Here's how the part is built. I have some questions about the finished solid (model axes, mm). Coordinates: 2 decimals unless noted, no trailing zeros. Write each loop counter-clockwise with the first axis right and the second up, starting at its lowest first coordinate (ties: lowest second). Pieces come first, ordered by that corner, then holes.
```python
from build123d import *

# Parameters (mm, degrees)
SKIZZE1_W                       = 8
SKIZZE1_H                       = 16
AUFSATZ_LINEAR_AUSTRAGEN1_DEPTH = 4.7
VERRUNDUNG1_R                   = 1
SKIZZE2_R                       = 3.5
SCHNITT_LINEAR_AUSTRAGEN1_DEPTH = 0.05


with BuildPart() as part:
    # Skizze1 → Aufsatz-Linear austragen1 (new body)
    with BuildSketch(Plane.XY):
        with Locations((4, -8)):
            Rectangle(SKIZZE1_W, SKIZZE1_H)
    extrude(amount=AUFSATZ_LINEAR_AUSTRAGEN1_DEPTH)

    # Verrundung1
    verrundung1_edges = [part.edges().sort_by_distance(p)[0] for p in [
        (0, 0, 2.35),
        (8, 0, 2.35),
        (8, -16, 2.35),
        (0, -16, 2.35),
    ]]
    fillet(verrundung1_edges, radius=VERRUNDUNG1_R)

    # Skizze2 → Schnitt-Linear austragen1 (cut)
    with BuildSketch(Plane.XY.offset(4.7)):
        with Locations((4, -4)):
            Circle(SKIZZE2_R)
    extrude(amount=-SCHNITT_LINEAR_AUSTRAGEN1_DEPTH, mode=Mode.SUBTRACT)

    # Skizze3 → Schnitt-Rotation1 (revolve, cut)
    with BuildSketch(Plane(origin=(4, 0, 0), x_dir=(0, 0, -1), z_dir=(1, 0, 0))):
        Polygon((-4.7, -8.75), (-3, -10.45), (0, -10.45), (0, -12), (-4.7, -12), align=None)
    revolve(axis=Axis((4, -12, 4.7), (0, 0, -1)), mode=Mode.SUBTRACT)


solid = part.part
```
1) Imagine slicing it at C-C on x = 4. Please give me the cut outline in (y, z), then the cut area to 3 significant figures.
Values follow:
outline: (-16, 0) - (-13.55, 0) - (-13.55, 3) - (-15.25, 4.7) - (-16, 4.7) - close; (-10.45, 0) - (0, 0) - (0, 4.7) - (-0.5, 4.7) - (-0.5, 4.65) - (-7.5, 4.65) - (-7.5, 4.7) - (-8.75, 4.7) - (-10.45, 3) - close
area: 57.4 mm2
2) Imagine slicing it at A-A on y = -12. Please give me the cut outline in (x, z), then the cut area to 3 significant figures.
Values follow:
outline: (0, 0) - (2.45, 0) - (2.45, 3) - (0.75, 4.7) - (0, 4.7) - close; (5.55, 0) - (8, 0) - (8, 4.7) - (7.25, 4.7) - (5.55, 3) - close
area: 20.1 mm2
3) Imagine slicing it at D-D on z = 3.2. Please give me the cut outline in (x, y), then the cut area to 3 significant figures.
Values follow:
outline: (0, -15) arc R1 ccw to (1, -16) - (7, -16) arc R1 ccw to (8, -15) - (8, -1) arc R1 ccw to (7, 0) - (1, 0) arc R1 ccw to (0, -1) - close; hole circle Ø3.5 at (4, -12)
area: 118 mm2
4) Will this pin go through, and if not, where does the flat tip stop? pin 1 (3.5 mm diameter, centred on x = 4, y = -12, fed in from +Z).
Values follow:
pin 1: stops at z = 3.2
5) I need wall thicknesses on probe 1 along X at (y, z) = (-12, 2.1); probe 2 along Z at (x, y) = (1.25, -2); probe 3 along Y at (x, z) = (2.75, 0.6). Which ranges of each line are inside material? Lowest first, please.
Values follow:
probe 1: x = 0 to 2.45, 5.55 to 8
probe 2: z = 0 to 4.65
probe 3: y = -16 to -12.92, -11.08 to 0
6) Imagine slicing it at B-B on z = 0.85. Please give me the cut outline in (x, y).
Values follow:
outline: (0, -15) arc R1 ccw to (1, -16) - (7, -16) arc R1 ccw to (8, -15) - (8, -1) arc R1 ccw to (7, 0) - (1, 0) arc R1 ccw to (0, -1) - close; hole circle Ø3.1 at (4, -12)
7) We'd pull the mould along Y, two halves only. Please class faces 1 (the face through (7.715, -0.301, 2.383)), 2 (the face through (4, -4, 4.65)), 3 (the face through (8, -8, 2)): pulls with the +Y half, pulls with the -Y half, needs draft (parallel to the pull), parting line crosses it, or undercut.
Values follow:
face 1: pulls with the +Y half
face 2: undercut
face 3: needs draft
